Check sheet for the modelled part. Datum: model origin and axes. Units: mm. A direction names the side the tool comes from. Coordinates: 2 decimals unless noted, no trailing zeros. Write each loop counter-clockwise with the first axis right and the second up, starting at its lowest first coordinate (ties: lowest second). Pieces come first, ordered by that corner, then holes. Notation, with made-up numbers: (82.25, 48) -> (134.25, 48) arc R11 ccw to (134.25, 64) -> close; hole circle Ø4 at (-26, 15.5). An arc over 180 degrees is marked (long way). Put each result on its own line as item: value.
```python
from build123d import *

# Parameters (mm, degrees)
PAD003_DEPTH    = 1.6
PAD004_DEPTH    = 1.6
POCKET002_DEPTH = 1.6
PAD005_DEPTH    = 1.6
SKETCH015_R     = 1
SKETCH015_R_2   = 1.75
POCKET004_DEPTH = 1.6
PAD019_DEPTH    = 6


with BuildPart() as part:
    # Sketch005 → Pad003 (new body)
    with BuildSketch(Plane.XY):
        with BuildLine():
            Line((-19.6, 18.1), (-19.6, -18.1))
            ThreePointArc((-19.6, -18.1), (-19.16066, -19.16066), (-18.1, -19.6))
            Line((-18.1, -19.6), (18.1, -19.6))
            ThreePointArc((18.1, -19.6), (19.16066, -19.16066), (19.6, -18.1))
            Line((19.6, -18.1), (19.6, 18.1))
            ThreePointArc((19.6, 18.1), (19.16066, 19.16066), (18.1, 19.6))
            Line((18.1, 19.6), (-18.1, 19.6))
            ThreePointArc((-18.1, 19.6), (-19.16066, 19.16066), (-19.6, 18.1))
        make_face()
    extrude(amount=PAD003_DEPTH)

    # Sketch006 (on Face9 of Pad003) → Pad004 (join)
    with BuildSketch(Plane(origin=(0, 0, 0), x_dir=(1, 0, 0), z_dir=(0, 0, -1))):
        with BuildLine():
            Line((-18.8, 17.3), (-18.8, -17.3))
            ThreePointArc((-18.8, -17.3), (-18.36066, -18.36066), (-17.3, -18.8))
            Line((-17.3, -18.8), (17.3, -18.8))
            ThreePointArc((17.3, -18.8), (18.36066, -18.36066), (18.8, -17.3))
            Line((18.8, -17.3), (18.8, 17.3))
            ThreePointArc((18.8, 17.3), (18.36066, 18.36066), (17.3, 18.8))
            Line((17.3, 18.8), (-17.3, 18.8))
            ThreePointArc((-17.3, 18.8), (-18.36066, 18.36066), (-18.8, 17.3))
        make_face()
    extrude(amount=PAD004_DEPTH)

    # Sketch007 (on Face19 of Pad004) → Pocket002 (cut)
    with BuildSketch(Plane(origin=(0, 0, -1.6), x_dir=(1, 0, 0), z_dir=(0, 0, -1))):
        with BuildLine():
            Line((-18, -16.5), (-18, 16.5))
            ThreePointArc((-16.5, 18), (-17.56066, 17.56066), (-18, 16.5))
            Line((-16.5, 18), (16.5, 18))
            ThreePointArc((18, 16.5), (17.56066, 17.56066), (16.5, 18))
            Line((18, 16.5), (18, -16.5))
            ThreePointArc((16.5, -18), (17.56066, -17.56066), (18, -16.5))
            Line((16.5, -18), (-16.5, -18))
            ThreePointArc((-18, -16.5), (-17.56066, -17.56066), (-16.5, -18))
        make_face()
    extrude(amount=-POCKET002_DEPTH, mode=Mode.SUBTRACT)

    # Sketch008 (on Face28 of Pocket002) → Pad005 (join)
    with BuildSketch(Plane(origin=(0, 0, 0), x_dir=(1, 0, 0), z_dir=(0, 0, -1))):
        with BuildLine():
            ThreePointArc((-18, -16.499999), (-17.560661, -17.56066), (-16.5, -18))
            Line((18, 16.5), (-16.5, -18))
            ThreePointArc((18, 16.5), (17.56066, 17.56066), (16.5, 18))
            Line((-18, -16.499999), (16.5, 18))
        make_face()
        with BuildLine():
            ThreePointArc((-16.5, 18), (-17.56066, 17.56066), (-18, 16.5))
            Line((-18, 16.5), (16.5, -18))
            ThreePointArc((16.5, -18), (17.56066, -17.56066), (18, -16.5))
            Line((-16.5, 18), (18, -16.5))
        make_face()
    extrude(amount=PAD005_DEPTH)

    # Sketch015 (on Face5 of Pad005) → Pocket004 (cut)
    with BuildSketch(Plane.XY.offset(1.6)):
        with Locations((-7.9, 12.85)):
            Circle(SKETCH015_R)
        with Locations((6.6, 12.85)):
            Circle(SKETCH015_R)
        with Locations((-12.85, 1)):
            Circle(SKETCH015_R_2)
    extrude(amount=-POCKET004_DEPTH, mode=Mode.SUBTRACT)

    # Sketch030 (on Face37 of Pocket004) → Pad019 (join)
    with BuildSketch(Plane(origin=(0, 0, -1.6), x_dir=(1, 0, 0), z_dir=(0, 0, -1))):
        with BuildLine():
            ThreePointArc((-16.5, 18), (-17.56066, 17.56066), (-18, 16.5))
            Line((-18, 16.5), (-14.464466, 12.964466))
            Line((-14.464466, 12.964466), (-12.964466, 14.464466))
            Line((-16.5, 18), (-12.964466, 14.464466))
        make_face()
        with BuildLine():
            ThreePointArc((18, 16.5), (17.56066, 17.56066), (16.5, 18))
            Line((16.5, 18), (12.964466, 14.464466))
            Line((12.964466, 14.464466), (14.464466, 12.964466))
            Line((18, 16.5), (14.464466, 12.964466))
        make_face()
        with BuildLine():
            ThreePointArc((16.5, -18), (17.56066, -17.56066), (18, -16.5))
            Line((18, -16.5), (14.464466, -12.964466))
            Line((14.464466, -12.964466), (12.964466, -14.464466))
            Line((16.5, -18), (12.964466, -14.464466))
        make_face()
        with BuildLine():
            ThreePointArc((-18, -16.499999), (-17.56066, -17.56066), (-16.5, -18))
            Line((-16.5, -18), (-12.964466, -14.464466))
            Line((-14.464466, -12.964465), (-12.964466, -14.464466))
            Line((-18, -16.499999), (-14.464466, -12.964465))
        make_face()
    extrude(amount=PAD019_DEPTH)


with BuildPart() as part_1:
    # Body001 placement: moved
    add(part.part.moved(Location((0, 0, 13.2))))


solid = part_1.part
```
Q1. Material ranges on line 1 along Y through (x, z) = (6.6, 13.8); line 2 along Y through (x, z) = (16, 12.75); line 3 along Z through (x, y) = (-2, -16), recorded low to high.
Recorded:
line 1: y = -19.6 to 11.85, 13.85 to 19.6
line 2: y = -18.8 to -18, -17.5 to -14.5, 14.5 to 17.5, 18 to 18.8
line 3: z = 13.2 to 14.8
Q2. Cross-section at C-C (z = 12.25). Record the cut outline in (x, y), plus the area to 3 significant figures.
Recorded:
outline: (-18.8, -17.3) arc R1.5 ccw to (-17.3, -18.8) -> (17.3, -18.8) arc R1.5 ccw to (18.8, -17.3) -> (18.8, 17.3) arc R1.5 ccw to (17.3, 18.8) -> (-17.3, 18.8) arc R1.5 ccw to (-18.8, 17.3) -> close; hole (-18, -16.5) -> (-1.5, 0) -> (-18, 16.5) -> close; hole (-16.5, -18) -> (16.5, -18) -> (0, -1.5) -> close; hole (-16.5, 18) -> (0, 1.5) -> (16.5, 18) -> close; hole (1.5, 0) -> (18, -16.5) -> (18, 16.5) -> close
area: 323 mm2
Q3. Tool access check on faces 4 (the flat face through (12, 0, 13.2)), 5 (the flat face through (0, 18.8, 12)), 6 (the cylindrical face through (19.17, 19.15, 13.99)), 7 (the flat face through (-18.8, 0, 12)), 8 (the flat face through (-16, -16, 5.6)). Record the directions out of +Z, -Z, +X, -X, +Y, -Y that give a thin tool (end or side, any length) a straight path to the whole face; none if there is none.
Recorded:
face 4: -Z
face 5: -Z, +X, -X, +Y
face 6: +Z, -Z, +X, +Y
face 7: -Z, -X, +Y, -Y
face 8: -Z, +X, -X, +Y, -Y
Q4. Cross-section at D-D (z = 10.25). Record the cut outline in (x, y).
Recorded:
outline: (-18, -16.5) arc R1.5 ccw to (-16.5, -18) -> (-12.96, -14.46) -> (-14.46, -12.96) -> close; (-18, 16.5) -> (-14.46, 12.96) -> (-12.96, 14.46) -> (-16.5, 18) arc R1.5 ccw to start; (12.96, -14.46) -> (16.5, -18) arc R1.5 ccw to (18, -16.5) -> (14.46, -12.96) -> close; (12.96, 14.46) -> (14.46, 12.96) -> (18, 16.5) arc R1.5 ccw to (16.5, 18) -> close
Q5. Cross-section at B-B (x = 6.6). Record the cut outline in (y, z), plus the area to 3 significant figures.
Recorded:
outline: (-19.6, 13.2) -> (-18.8, 13.2) -> (-18.8, 11.6) -> (-18, 11.6) -> (-18, 13.2) -> (-8.1, 13.2) -> (-8.1, 11.6) -> (-5.1, 11.6) -> (-5.1, 13.2) -> (5.1, 13.2) -> (5.1, 11.6) -> (8.1, 11.6) -> (8.1, 13.2) -> (11.85, 13.2) -> (11.85, 14.8) -> (-19.6, 14.8) -> close; (13.85, 13.2) -> (18, 13.2) -> (18, 11.6) -> (18.8, 11.6) -> (18.8, 13.2) -> (19.6, 13.2) -> (19.6, 14.8) -> (13.85, 14.8) -> close
area: 71.7 mm2
Q6. Mould release check, pull along X, two halves, no side actions. Record for faces 1 (the cylindrical face through (-17.57, 17.55, 8.64)), 2 (the cylindrical face through (18.37, -18.35, 12.41)), 3 (the flat face through (-12, 13.5, 12)): released by +X, released by -X, zero draft, split by the parting line, or undercut.
Recorded:
face 1: released by -X
face 2: released by +X
face 3: undercut
Q7. Depth check by flat-ended pin: P1, Ø0.5, axis at y = -7, z = 12.5, coming from the -X side; P2, Ø3, axis at x = -2, y = 15, coming from the -Z side; P3, Ø23, axis at x = 6, y = 4.5, coming from the -Z side; P4, Ø3, axis at x = -12.85, y = 1, coming from the +Z side. Enter the tip coordinate at first touch or a pass-through.
Recorded:
P1: stops at x = -18.8
P2: stops at z = 13.2
P3: stops at z = 11.6
P4: passes through
Q8. Cross-section at A-A (y = 1). Record the cut outline in (x, z), plus the area to 3 significant figures.
Recorded:
outline: (-19.6, 13.2) -> (-18.8, 13.2) -> (-18.8, 11.6) -> (-18, 11.6) -> (-18, 13.2) -> (-14.6, 13.2) -> (-14.6, 14.8) -> (-19.6, 14.8) -> close; (-11.1, 13.2) -> (-2.5, 13.2) -> (-2.5, 11.6) -> (2.5, 11.6) -> (2.5, 13.2) -> (18, 13.2) -> (18, 11.6) -> (18.8, 11.6) -> (18.8, 13.2) -> (19.6, 13.2) -> (19.6, 14.8) -> (-11.1, 14.8) -> close
area: 67.7 mm2
